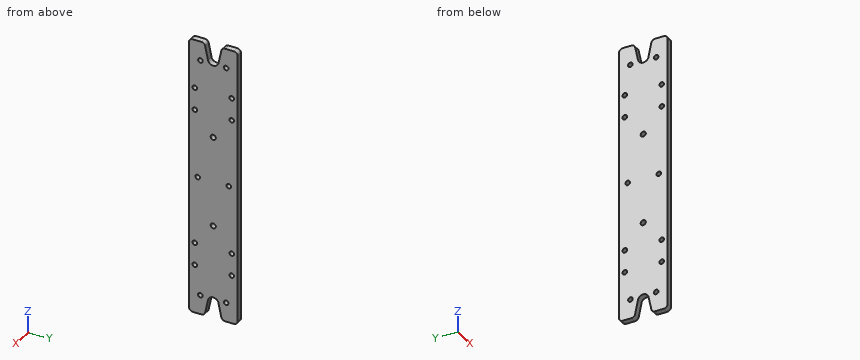
Autodesk Inventor part; units mm, degrees
ref_plane "YZ Plane" through (0, 0, 0) normal (1, 0, 0) x (0, 1, 0)
ref_plane "XZ Plane" through (0, 0, 0) normal (0, 1, 0) x (-1, 0, 0)
ref_plane "XY Plane" through (0, 0, 0) normal (0, 0, 1) x (1, 0, 0)
sketch "Sketch1" plane through (0, 0, 0) normal (1, 0, 0) x (0, 1, 0)
  line L0 (31.625, -180) -> (-31.625, -180)
  line L1 (-31.625, -180) -> (-31.625, 180)
  line L2 (-31.625, 180) -> (31.625, 180)
  line L3 (31.625, 180) -> (31.625, -180)
  line L4 (31.625, -180) -> (-31.625, 180) construction
  line L5 (-31.625, -180) -> (31.625, 180) construction
  line L6 (-31.625, 0) -> (31.625, 0) construction
  line L7 (0, 180) -> (0, -180) construction
  line L8 (24, -88) -> (-24, -88) construction
  line L9 (24, -117) -> (-24, -117) construction
  line L10 (16.75, -155) -> (-16.75, -155) construction
  line L11 (24, 88) -> (-24, 88) construction
  line L12 (24, 117) -> (-24, 117) construction
  line L13 (16.75, 155) -> (-16.75, 155) construction
  line L14 (24, -117) -> (24, -88) construction
  arc A0 (-6.8516, 158.566) -> (6.8516, 158.566) centre (0, 160) ccw
  line L15 (-15, 197.5) -> (15, 197.5)
  line L16 (15, 197.5) -> (6.8516, 158.566)
  line L17 (-15, 197.5) -> (-6.8516, 158.566)
  arc A1 (6.8516, -158.566) -> (-6.8516, -158.566) centre (0, -160) ccw
  line L18 (-15, -197.5) -> (15, -197.5)
  line L19 (15, -197.5) -> (6.8516, -158.566)
  line L20 (-15, -197.5) -> (-6.8516, -158.566)
  point P0 (0, 0)
  point P1 (-20.25, 0)
  point P2 (20.25, 0)
  point P3 (0, 155)
  point P4 (-11.3374, -180)
  point P5 (11.3374, -180)
  point P6 (11.3374, 180)
  point P7 (-11.3374, 180)
  point P8 (0, 58.5)
  point P9 (0, -58.5)
  dimension "d0" = 63.25
  dimension "d1" = 360
  dimension "d2" = 40.5
  dimension "d3" = 176
  dimension "d4" = 29
  dimension "d5" = 48
  dimension "d6" = 33.5
  dimension "d7" = 310
  dimension "d8" = 30
  dimension "d9" = 37.5
  dimension "d10" = 14
  dimension "d11" = 320
  dimension "d21" = 117
extrude "Extrusion1" add sketch "Sketch1" along normal blind 8 contours L0 L19 A1 L20 L1 L2 L17 A0 L16 L3
hole "Phi6-H7" at (0, -20.25, 0) at (0, 20.25, 0) at (0, 24, -88) at (0, 24, -117) at (0, 16.75, -155) at (0, -24, -88) at (0, -24, -117) at (0, -16.75, -155) at (0, 24, 88) at (0, 24, 117) at (0, 16.75, 155) at (0, -16.75, 155) at (0, -24, 117) at (0, -24, 88) at (0, 0, 160) at (0, 0, -160) direction (1, 0, 0) diameter 6 end through all
hole "M8" at (0, 0, 58.5) at (0, 0, -58.5) direction (1, 0, 0) diameter 6.647 end through all
fillet "R5" radius 5 8 edges at (4, 31.625, 180) (4, -31.625, 180) (4, 31.625, -180) (4, 11.3374, -180) (4, -11.3374, -180) (4, -31.625, -180) (4, -11.3374, 180) (4, 11.3374, 180)
properties part number "InitialPositioningFrame" material "Aluminum 7075"
Work out the finished part from the listing and answer in its coordinate system (mm). Give positions to 0.01 mm unless a question says otherwise; leave off trailing zeros. Loops run counter-clockwise (first coordinate to the right, second up) from the corner with the lowest first, then second, coordinate; pieces in that order, holes last. Notation, with made-up numbers: (22.25, 59) - (32.25, 59) arc R20 ccw to (32.25, 83) - close; hole circle Ø10 at (16.5, -4). An arc over 180 degrees is marked (long way). One line per question, with ' | ' between items.
(1) The part is cut by section D-D (x = 5.25). Count the separate pieces of the cut face and the enclosed holes in it, then the cut area to 3 significant figures.
Recorded:
separate pieces: 1 | enclosed holes: 16 | area: 21,400 mm²
(2) The part is cut by section C-C (z = 58.5). Write down the section's boundary in (x, y) (1 decimal).
Recorded:
outline: (0, -31.6) - (8, -31.6) - (8, -3.3) - (0, -3.3) - close; (0, 3.3) - (8, 3.3) - (8, 31.6) - (0, 31.6) - close
(3) The part is cut by section A-A (z = -88). Write down the section's boundary in (x, y) (3 decimals), then the cut area to 3 significant figures.
Recorded:
outline: (0, -31.625) - (8, -31.625) - (8, -27) - (0, -27) - close; (0, -21) - (8, -21) - (8, 21) - (0, 21) - close; (0, 27) - (8, 27) - (8, 31.625) - (0, 31.625) - close | area: 410 mm²
(4) Straight lines are drawn through the part: probe 1 along Y at (x, z) = (2.5, -88) (3 decimals); probe 2 along Z at (x, y) = (5.5, -24); probe 3 along Y at (x, z) = (3, -58.5) (1 decimal). For each, find the intervals that lie inside material, in ascending order.
Recorded:
probe 1: y = -31.625 to -27, -21 to 21, 27 to 31.625 | probe 2: z = -180 to -120, -114 to -91, -85 to 85, 91 to 114, 120 to 180 | probe 3: y = -31.6 to -3.3, 3.3 to 31.6
(5) The part is cut by section B-B (y = 0). Write down the section's boundary in (x, z).
Recorded:
outline: (0, -153) - (8, -153) - (8, -61.82) - (0, -61.82) - close; (0, -55.18) - (8, -55.18) - (8, 55.18) - (0, 55.18) - close; (0, 61.82) - (8, 61.82) - (8, 153) - (0, 153) - close
(6) This flat-tipped pin is pushed along its axis until it touches: pin 1 Ø3 at (x, y) = (2, 4.5) entering from +Z. Where does it stop, or does it pass through?
Recorded:
pin 1: stops at z = 156.39
